```python
from build123d import *

# Parameters (mm, degrees)
SKETCH1_W            = 39
SKETCH1_H            = 49.22
BOSS_EXTRUDE2_DEPTH  = 30
SKETCH3_W            = 1.75
SKETCH3_H            = 20
SKETCH3_W_2          = 1
SKETCH3_H_2          = 15.1
CUT_EXTRUDE3_DEPTH   = 47.22
CUT_EXTRUDE4_DEPTH   = 47.22
CUT_EXTRUDE5_DEPTH   = 3.75
SKETCH9_W            = 22.2
SKETCH9_H            = 30
CUT_EXTRUDE7_DEPTH   = 61.922592565
SKETCH11_W           = 0.8
SKETCH11_H           = 21.811754546
SKETCH11_H_2         = 8.188245454
CUT_EXTRUDE8_DEPTH   = 46.008146799
SKETCH12_W           = 23
SKETCH12_H           = 2.5
BOSS_EXTRUDE3_DEPTH  = 3
SKETCH13_W           = 23
SKETCH13_H           = 2.5
BOSS_EXTRUDE4_DEPTH  = 3
BOSS_EXTRUDE5_REACH  = 51.909
SKETCH14_W           = 27.02
SKETCH14_H           = 3
SKETCH15_W           = 30.25
SKETCH15_H           = 3
CUT_EXTRUDE9_DEPTH   = 25.02
SKETCH16_W           = 30.25
SKETCH16_H           = 3
CUT_EXTRUDE10_DEPTH  = 46.276919382
SKETCH24_W           = 23
SKETCH24_H           = 2.5
BOSS_EXTRUDE8_DEPTH  = 6
BOSS_EXTRUDE9_DEPTH  = 3
SKETCH26_W           = 41.2
SKETCH26_H           = 27.02
BOSS_EXTRUDE10_DEPTH = 3
SKETCH29_W           = 4.264424859
SKETCH29_H           = 26.447816837
CUT_EXTRUDE14_DEPTH  = 41.905994632
SKETCH30_W           = 3.981396999
SKETCH30_H           = 33.655588154
CUT_EXTRUDE15_DEPTH  = 40.425282457
BOSS_EXTRUDE15_DEPTH = 2
BOSS_EXTRUDE16_DEPTH = 2
SKETCH36_W           = 41.2
SKETCH36_H           = 4.993514727
BOSS_EXTRUDE17_DEPTH = 26
SKETCH37_W           = 41.2
SKETCH37_H           = 5
BOSS_EXTRUDE18_DEPTH = 28.006485273
SKETCH38_W           = 41.2
SKETCH38_H           = 5
BOSS_EXTRUDE19_DEPTH = 20
BOSS_EXTRUDE21_DEPTH = 5
SKETCH40_R           = 2
CUT_EXTRUDE16_DEPTH  = 78.060934741
FILLET1_R            = 2
BOSS_EXTRUDE22_DEPTH = 10


with BuildPart() as part:
    # Sketch1 → Boss-Extrude2 (new body)
    with BuildSketch(Plane(origin=(0, 0, 0), x_dir=(1, 0, 0), z_dir=(0, 1, 0))):
        with Locations((-0.391025069, -11.314396792)):
            Rectangle(SKETCH1_W, SKETCH1_H)
    extrude(amount=BOSS_EXTRUDE2_DEPTH)

    # Sketch3 → Cut-Extrude3 (cut)
    with BuildSketch(Plane.XY.offset(35.924396792)):
        Polygon((16.108974931, 23.05), (16.108974931, 28), (-16.141025069, 28), (-16.141025069, 25.5), (-16.141025069, 5.5), (-16.141025069, 0), (16.108974931, 0), (16.108974931, 7.95), align=None)
        with Locations((-17.016025069, 15.5)):
            Rectangle(SKETCH3_W, SKETCH3_H)
        with Locations((16.608974931, 15.5)):
            Rectangle(SKETCH3_W_2, SKETCH3_H_2)
    extrude(amount=-CUT_EXTRUDE3_DEPTH, mode=Mode.SUBTRACT)

    # Sketch7 → Cut-Extrude4 (cut)
    with BuildSketch(Plane.ZY.offset(19.891025069)):
        with BuildLine():
            ThreePointArc((11.724396792, 15), (24.324396792, 2.4), (36.924396792, 15))
            ThreePointArc((36.924396792, 15), (24.324396792, 27.6), (11.724396792, 15))
        make_face()
    extrude(amount=-CUT_EXTRUDE4_DEPTH, mode=Mode.SUBTRACT)

    # Sketch8 → Cut-Extrude5 (cut)
    with BuildSketch(Plane.ZY.offset(19.891025069)):
        with BuildLine():
            Line((35.924396792, 30), (17.633933867, 30))
            Line((17.633933867, 30), (17.633933867, 27))
            Line((17.633933867, 27), (8.633933867, 27))
            Line((8.633933867, 27), (8.633933867, 4))
            Line((8.633933867, 4), (17.633933867, 4))
            Line((17.633933867, 4), (17.633933867, 0))
            Line((17.633933867, 0), (35.924396792, 0))
            Line((35.924396792, 0), (35.924396792, 10.08065045))
            ThreePointArc((35.924396792, 10.08065045), (11.724396792, 15), (35.924396792, 19.91934955))
            Line((35.924396792, 19.91934955), (35.924396792, 30))
        make_face()
    extrude(amount=-CUT_EXTRUDE5_DEPTH, mode=Mode.SUBTRACT)

    # Sketch9 → Cut-Extrude7 (cut, through all)
    with BuildSketch(Plane(origin=(19.108974931, 0, 0), x_dir=(0, 0, -1), z_dir=(1, 0, 0))):
        with Locations((-24.824396792, 15)):
            Rectangle(SKETCH9_W, SKETCH9_H)
    extrude(amount=-CUT_EXTRUDE7_DEPTH, mode=Mode.SUBTRACT)

    # Sketch11 → Cut-Extrude8 (cut, through all)
    with BuildSketch(Plane.XY.offset(13.724396792)):
        with Locations((18.708974931, 19.094122727)):
            Rectangle(SKETCH11_W, SKETCH11_H)
        with Locations((18.708974931, 4.094122727)):
            Rectangle(SKETCH11_W, SKETCH11_H_2)
    extrude(amount=-CUT_EXTRUDE8_DEPTH, mode=Mode.SUBTRACT)

    # Sketch12 → Boss-Extrude3 (add)
    with BuildSketch(Plane(origin=(18.308974931, 0, 0), x_dir=(0, 0, -1), z_dir=(1, 0, 0))):
        with Locations((1.795603208, 1.25)):
            Rectangle(SKETCH12_W, SKETCH12_H)
    extrude(amount=BOSS_EXTRUDE3_DEPTH)

    # Sketch13 → Boss-Extrude4 (add)
    with BuildSketch(Plane.ZY.offset(19.891025069)):
        with Locations((-1.795603208, 1.25)):
            Rectangle(SKETCH13_W, SKETCH13_H)
    extrude(amount=BOSS_EXTRUDE4_DEPTH)

    # Sketch14 → Boss-Extrude5 (add, up to next)
    with BuildSketch(Plane(origin=(-16.141025069, 0, 0), x_dir=(0, 0, -1), z_dir=(1, 0, 0)), mode=Mode.PRIVATE) as boss_extrude5_sk1:
        with Locations((-0.214396792, 1.5)):
            Rectangle(SKETCH14_W, SKETCH14_H)
    boss_extrude5_tool1 = extrude(boss_extrude5_sk1.sketch, amount=BOSS_EXTRUDE5_REACH, mode=Mode.PRIVATE) - part.part
    add(boss_extrude5_tool1.solids().sort_by_distance((-16.141025, 1.5, 0.214397))[0])

    # Sketch15 → Cut-Extrude9 (cut)
    with BuildSketch(Plane.XY.offset(13.724396792)):
        with Locations((-0.016025069, 1.5)):
            Rectangle(SKETCH15_W, SKETCH15_H)
    extrude(amount=-CUT_EXTRUDE9_DEPTH, mode=Mode.SUBTRACT)

    # Sketch16 → Cut-Extrude10 (cut, through all)
    with BuildSketch(Plane.XY.offset(-11.295603208)):
        with Locations((-0.016025069, 1.5)):
            Rectangle(SKETCH16_W, SKETCH16_H)
    extrude(amount=-CUT_EXTRUDE10_DEPTH, mode=Mode.SUBTRACT)

    # Sketch24 → Boss-Extrude8 (add)
    with BuildSketch(Plane.ZY.offset(22.891025069)):
        with Locations((-1.795603208, 1.25)):
            Rectangle(SKETCH24_W, SKETCH24_H)
    extrude(amount=BOSS_EXTRUDE8_DEPTH)

    # Sketch25 → Boss-Extrude9 (add)
    with BuildSketch(Plane.ZY.offset(19.891025069)):
        Polygon((-13.295603208, 30), (13.724396792, 30), (13.724396792, 27), (8.633933867, 27), (8.633933867, 4), (13.724396792, 4), (13.724396792, 0), (9.704396792, 0), (9.704396792, 2.5), (-13.295603208, 2.5), align=None)
    extrude(amount=BOSS_EXTRUDE9_DEPTH)

    # Sketch26 → Boss-Extrude10 (add)
    with BuildSketch(Plane(origin=(0, 30, 0), x_dir=(1, 0, 0), z_dir=(0, 1, 0))):
        with Locations((-2.291025069, -0.214396792)):
            Rectangle(SKETCH26_W, SKETCH26_H)
    extrude(amount=BOSS_EXTRUDE10_DEPTH)

    # Sketch29 → Cut-Extrude14 (cut, through all)
    with BuildSketch(Plane.XZ.offset(-25.5)):
        with Locations((-15.75881264, 1.92830521)):
            Rectangle(SKETCH29_W, SKETCH29_H)
    extrude(amount=CUT_EXTRUDE14_DEPTH, mode=Mode.SUBTRACT)

    # Sketch30 → Cut-Extrude15 (cut, through all)
    with BuildSketch(Plane(origin=(0, 23.05, 0), x_dir=(-1, 0, 0), z_dir=(0, -1, 0))):
        with Locations((-15.118276432, -5.532190869)):
            Rectangle(SKETCH30_W, SKETCH30_H)
    extrude(amount=CUT_EXTRUDE15_DEPTH, mode=Mode.SUBTRACT)

    # Sketch34 → Boss-Extrude15 (add)
    with BuildSketch(Plane(origin=(0, 0, -13.295603208), x_dir=(-1, 0, 0), z_dir=(0, 0, -1))):
        Polygon((-18.308974931, 33), (-18.308974931, 2.5), (-21.308974931, 2.5), (-21.308974931, 0), (28.891025069, 0), (28.891025069, 2.5), (22.891025069, 2.5), (22.891025069, 33), align=None)
    extrude(amount=-BOSS_EXTRUDE15_DEPTH)

    # Sketch35 → Boss-Extrude16 (add)
    with BuildSketch(Plane(origin=(0, 0, -13.295603208), x_dir=(-1, 0, 0), z_dir=(0, 0, -1))):
        Polygon((-18.308974931, 33), (-18.308974931, 2.5), (-21.308974931, 2.5), (-21.308974931, 0), (28.891025069, 0), (28.891025069, 2.5), (22.891025069, 2.5), (22.891025069, 33), align=None)
    extrude(amount=BOSS_EXTRUDE16_DEPTH)

    # Sketch36 → Boss-Extrude17 (add)
    with BuildSketch(Plane.XY.offset(13.724396792)):
        with Locations((-2.291025069, 30.503242637)):
            Rectangle(SKETCH36_W, SKETCH36_H)
    extrude(amount=BOSS_EXTRUDE17_DEPTH)

    # Sketch37 → Boss-Extrude18 (add)
    with BuildSketch(Plane(origin=(0, 28.006485273, 0), x_dir=(-1, 0, 0), z_dir=(0, -1, 0))):
        with Locations((2.291025069, -37.224396792)):
            Rectangle(SKETCH37_W, SKETCH37_H)
    extrude(amount=BOSS_EXTRUDE18_DEPTH)

    # Sketch38 → Boss-Extrude19 (add)
    with BuildSketch(Plane.XY.offset(39.724396792)):
        with Locations((-2.291025069, 2.5)):
            Rectangle(SKETCH38_W, SKETCH38_H)
    extrude(amount=BOSS_EXTRUDE19_DEPTH)

    # Sketch39 → Boss-Extrude21 (add)
    with BuildSketch(Plane(origin=(0, 5, 0), x_dir=(1, 0, 0), z_dir=(0, 1, 0))):
        with BuildLine():
            Line((-8.291025069, -59.724396792), (-22.891025069, -59.724396792))
            Line((-22.891025069, -59.724396792), (-4.038597885, -65.464256481))
            ThreePointArc((-4.038597885, -65.464256481), (-7.112095329, -63.296130482), (-8.291025069, -59.724396792))
        make_face()
        with BuildLine():
            ThreePointArc((-8.291025069, -59.724396792), (-7.112095329, -63.296130482), (-4.038597885, -65.464256481))
            ThreePointArc((-4.038597885, -65.464256481), (-2.291025069, -65.724396792), (-0.543452254, -65.464256481))
            ThreePointArc((-0.543452254, -65.464256481), (2.53004519, -63.296130482), (3.708974931, -59.724396792))
            Line((3.708974931, -59.724396792), (-0.291025069, -59.724396792))
            ThreePointArc((-0.291025069, -59.724396792), (-2.291025069, -61.724396792), (-4.291025069, -59.724396792))
            Line((-4.291025069, -59.724396792), (-8.291025069, -59.724396792))
        make_face()
        with BuildLine():
            ThreePointArc((3.708974931, -59.724396792), (-2.291025069, -53.724396792), (-8.291025069, -59.724396792))
            Line((-8.291025069, -59.724396792), (-4.291025069, -59.724396792))
            ThreePointArc((-4.291025069, -59.724396792), (-2.291025069, -57.724396792), (-0.291025069, -59.724396792))
            Line((-0.291025069, -59.724396792), (3.708974931, -59.724396792))
        make_face()
        with BuildLine():
            ThreePointArc((3.708974931, -59.724396792), (2.53004519, -63.296130482), (-0.543452254, -65.464256481))
            Line((-0.543452254, -65.464256481), (18.308974931, -59.724396792))
            Line((18.308974931, -59.724396792), (3.708974931, -59.724396792))
        make_face()
    extrude(amount=-BOSS_EXTRUDE21_DEPTH)

    # Sketch40 → Cut-Extrude16 (cut, through all)
    with BuildSketch(Plane(origin=(0, 5, 0), x_dir=(1, 0, 0), z_dir=(0, 1, 0))):
        with Locations(Location((-2.291025069, -59.724396792, 0), (0, 0, 270))):
            Circle(SKETCH40_R)
    extrude(amount=-CUT_EXTRUDE16_DEPTH, mode=Mode.SUBTRACT)

    # Fillet1
    fillet1_edges = [part.edges().sort_by_distance(p)[0] for p in [
        (-22.891025069, 33, 12.214396792),
        (18.308974931, 33, 12.214396792),
        (-2.291025069, 33, -15.295603208),
        (-2.291025069, 33, 39.724396792),
        (-22.891025069, 2.5, 59.724396792),
        (18.308974931, 2.5, 59.724396792),
    ]]
    fillet(fillet1_edges, radius=FILLET1_R)

    # Sketch41 → Boss-Extrude22 (add)
    with BuildSketch(Plane(origin=(0, 0, -15.295603208), x_dir=(-1, 0, 0), z_dir=(0, 0, -1))):
        Polygon((17.291025069, 5), (2.291025069, 5), (-12.708974931, 5), (-12.708974931, 0), (2.291025069, 0), (17.291025069, 0), align=None)
    extrude(amount=BOSS_EXTRUDE22_DEPTH)


solid = part.part
```
Geometry check sheet. Reference: the model listing, model coordinates, mm. A direction names the side the tool comes from. Coordinates: 2 decimals unless noted, no trailing zeros. Order: outer loops, then holes, each group sorted by start corner. A loop starts at its lowest first (then second) coordinate and runs counter-clockwise, first axis right, second up.
Q1. Sectioned sample at B-B on z = 3. Record the cut outline in (x, y), and give its area (3 significant figures).
Reply:
outline: (-28.89, 0) - (-17.89, 0) - (-17.89, 25.5) - (-16.14, 25.5) - (-16.14, 28) - (16.11, 28) - (16.11, 23.05) - (17.11, 23.05) - (17.11, 0) - (21.31, 0) - (21.31, 2.5) - (18.31, 2.5) - (18.31, 31) arc R2 ccw to (16.31, 33) - (-20.89, 33) arc R2 ccw to (-22.89, 31) - (-22.89, 2.5) - (-28.89, 2.5) - close
area: 410 mm2
Q2. Tool access check on faces 1 (the face through (12.709, 3, -20)), 2 (the face through (-17, 25.5, -1)), 3 (the face through (-3, 28.006, 24)), 4 (the face through (20, 2.5, -3)). Record the directions out of +Z, -Z, +X, -X, +Y, -Y that give a thin tool (end or side, any length) a straight path to the whole face; none if there is none.
Reply:
face 1: -Z, +X, +Y, -Y
face 2: -Y
face 3: +X, -X, -Y
face 4: +Z, -Z, +X, +Y
Q3. Depth check by flat-ended pin: pin 1 Ø8 at (y, z) = (10, -0.5) entering from -X; pin 2 Ø4.5 at (x, z) = (-2.29, 59.72) entering from +Y; pin 3 Ø1.5 at (x, z) = (20, -1.5) entering from +Y. Enter the tip coordinate at first touch or a pass-through.
Reply:
pin 1: stops at x = -22.89
pin 2: stops at y = 5
pin 3: stops at y = 2.5
Q4. Draft check along Z on faces 5 (the face through (17.701, 15.101, 11.725)), 6 (the face through (-28.891, 1, -3)), 7 (the face through (-12.878, 2.535, 62.773)). Enter one of: released by +Z, released by -Z, zero draft, split by the parting line, or undercut.
Reply:
face 5: undercut
face 6: zero draft
face 7: released by +Z
Q5. Sectioned sample at A-A on y = 24. Record the cut outline in (x, z), and give its area (3 significant figures).
Reply:
outline: (-22.89, -15.3) - (18.31, -15.3) - (18.31, 13.72) - (16.11, 13.72) - (16.11, -11.3) - (-17.89, -11.3) - (-17.89, 8.63) - (-22.89, 8.63) - close; (-22.89, 34.72) - (18.31, 34.72) - (18.31, 39.72) - (-22.89, 39.72) - close
area: 525 mm2
Q6. Sectioned sample at D-D on y = 12. Record the cut outline in (x, z), and give its area (3 significant figures).
Reply:
outline: (-22.89, -15.3) - (18.31, -15.3) - (18.31, 12.09) - (17.11, 12.09) - (17.11, -11.3) - (-17.89, -11.3) - (-17.89, 8.63) - (-22.89, 8.63) - close; (-22.89, 34.72) - (18.31, 34.72) - (18.31, 39.72) - (-22.89, 39.72) - close
area: 499 mm2
Q7. Thickness scan on probe 1 along X at (y, z) = (20, 8.5); probe 2 along Z at (x, y) = (18, 15); probe 3 along Z at (x, y) = (6, 27). Record the ranges inside material, lowest first.
Reply:
probe 1: x = -22.89 to -17.89, 17.11 to 18.31
probe 2: z = -15.3 to 11.72, 34.72 to 39.72
probe 3: z = -15.3 to -11.3, 34.72 to 39.72
